Read the model definition and answer for the solid it produces. Units are mm, in the model's axes. A direction names the side the tool comes from. Coordinates: 2 decimals unless noted, no trailing zeros. Loops run counter-clockwise (first coordinate to the right, second up) from the corner with the lowest first, then second, coordinate; pieces in that order, holes last. Notation, with made-up numbers: M -40,64 L -18,64 A8 ccw -18,73 Z; hole C 47.25,87 d6. An arc over 180 degrees is marked long. Put each result on its own line as item: value.
from build123d import *

# Parameters (mm, degrees)
BOSS_EXTRUDE1_DEPTH = 11.176
CHAMFER1_SIZE       = 0.254


with BuildPart() as part:
    # Sketch2 → Revolve1 (revolve)
    with BuildSketch(Plane.XY, mode=Mode.PRIVATE) as revolve1_sk:
        Polygon((0, 0), (0, 16.2941), (1.27, 16.2941), (1.27, 11.2141), (5.5245, 14.224), (5.5245, 16.764), (8.6995, 16.764), (8.6995, 10.033), (10.4521, 8.2804), (10.4521, 4.2926), (8.6995, 2.54), (8.6995, 0), align=None)
    revolve(revolve1_sk.sketch.rotate(Axis((0, 0, 0), (0, 1, 0)), 90), axis=Axis((0, 0, 0), (0, 1, 0)))

    # Sketch3 → Boss-Extrude1 (add)
    with BuildSketch(Plane.XZ):
        Polygon((13.931461996, 0), (6.965730998, 12.065), (-6.965730998, 12.065), (-13.931461996, 0), (-6.965730998, -12.065), (6.965730998, -12.065), align=None)
    extrude(amount=BOSS_EXTRUDE1_DEPTH)

    # Sketch5 → Cut-Revolve1 (revolve, cut)
    with BuildSketch(Plane.XY, mode=Mode.PRIVATE) as cut_revolve1_sk:
        Polygon((13.931461996, -1.778), (12.153461996, 0), (16.589687484, 0), (16.589687484, -11.176), (12.153461996, -11.176), (13.931461996, -9.398), align=None)
    revolve(cut_revolve1_sk.sketch.rotate(Axis((0, 0, 0), (0, -1, 0)), 90), axis=Axis((0, 0, 0), (0, -1, 0)), mode=Mode.SUBTRACT)

    # Chamfer1
    chamfer1_edges = [part.edges().sort_by_distance(p)[0] for p in [
        (0, 16.764, 8.6995),
        (0, 0, 8.6995),
    ]]
    chamfer(chamfer1_edges, length=CHAMFER1_SIZE)


solid = part.part
1) Which of the six approach directions +Z, -Z, +X, -X, +Y, -Y give full straight-line access (tool end or side, diameter ignored) to faces 1 (the flat face through (10.497, -5.51, 5.948)), 2 (the cylindrical face through (4.003, 6.259, -9.655))?
Answer list:
face 1: +Z, +X, +Y, -Y
face 2: +Y
2) Find section B-B, the plane y = -6.75. Write down the section's boundary in (x, z) (3 decimals).
Answer list:
outline: M -13.931,0 L -6.966,-12.065 L 6.966,-12.065 L 13.931,0 L 6.966,12.065 L -6.966,12.065 Z
3) Find section C-C, the plane y = -0.75. Write down the section's boundary in (x, z) (3 decimals).
Answer list:
outline: M -12.736,-2.07 L -8.161,-9.995 A12.903 ccw -4.575,-12.065 L 4.575,-12.065 A12.903 ccw 8.161,-9.995 L 12.736,-2.07 A12.903 ccw 12.736,2.07 L 8.161,9.995 A12.903 ccw 4.575,12.065 L -4.575,12.065 A12.903 ccw -8.161,9.995 L -12.736,2.07 A12.903 ccw Z
4) Determine the mould class of faces 3 (the conical face through (6.27, -10.67, -11)), 4 (the conical face through (6.256, -0.481, -10.978)), 5 (the flat face through (-9.1, 0, -0.8)), 6 (the flat face through (-10.4, -5.51, 6.12)) for opening direction Y: released by +Y, released by -Y, zero draft, split by the parting line, or undercut.
Answer list:
face 3: released by -Y
face 4: released by +Y
face 5: undercut
face 6: zero draft
5) Given pin 1 Ø6 at (y, z) = (10, 8.5) entering from +X; pin 2 Ø1 at (y, z) = (13.5, 4.5) entering from -X; pin 3 Ø4 at (x, z) = (9.5, -7.5) entering from +Y; pin 4 Ø12 at (x, y) = (6.5, 4) entering from +Z (3 decimals), each flat-ended and moving along its own axis, determine where each tip first touches the part or whether it passes through.
Answer list:
pin 1: stops at x = 8.53
pin 2: stops at x = -7.73
pin 3: stops at y = 8.63
pin 4: stops at z = 12.065
6) Straight lines are drawn through the part: line 1 (X direction, y = 15.95, z = 0); line 2 (Z direction, x = 0.25, y = 12.25); line 3 (Y direction, x = 9.5, z = -6.25). For each, find the intervals that lie inside material, in ascending order. Write a range as [from, to].
Answer list:
line 1: x = [-8.7, -5.52], [-1.27, 1.27], [5.52, 8.7]
line 2: z = [-8.7, -2.72], [-1.25, 1.25], [2.72, 8.7]
line 3: y = [-11.18, 0]
7) Find section D-D, the plane y = 5.75. Write down the section's boundary in (x, z).
Answer list:
outline: C 0,0 d20.9
